from build123d import *

# Parameters (mm, degrees)
CROQUIS1_R              = 3.125
CROQUIS1_R_2            = 2.7
SALIENTE_EXTRUIR1_DEPTH = 10
CROQUIS2_W              = 22
CROQUIS2_H              = 15
SALIENTE_EXTRUIR2_DEPTH = 50
CROQUIS3_R              = 4
CORTAR_EXTRUIR1_DEPTH   = 63.841873384


with BuildPart() as part:
    # Croquis1 → Saliente-Extruir1 (new body)
    with BuildSketch(Plane.XY):
        with Locations((0.140065102, 8.039289834)):
            Circle(CROQUIS1_R)
        with Locations((0.140065102, 8.039289834)):
            Circle(CROQUIS1_R_2, mode=Mode.SUBTRACT)
    extrude(amount=SALIENTE_EXTRUIR1_DEPTH)

    # Croquis2 → Saliente-Extruir2 (add)
    with BuildSketch(Plane.XY.offset(10)):
        with Locations((0.140065102, 8.039289834)):
            Rectangle(CROQUIS2_W, CROQUIS2_H)
    extrude(amount=SALIENTE_EXTRUIR2_DEPTH)

    # Croquis3 → Cortar-Extruir1 (cut, through all)
    with BuildSketch(Plane.XZ.offset(-0.539289834)):
        with Locations(Location((0.140065102, 35, 0), (0, 0, 270))):
            Circle(CROQUIS3_R)
    extrude(amount=-CORTAR_EXTRUIR1_DEPTH, mode=Mode.SUBTRACT)


solid = part.part
Geometry check sheet. Reference: the model listing, model coordinates, mm. A direction names the side the tool comes from. Coordinates: 2 decimals unless noted, no trailing zeros. Order: outer loops, then holes, each group sorted by start corner. A loop starts at its lowest first (then second) coordinate and runs counter-clockwise, first axis right, second up. Notation, with made-up numbers: (44.5, 39) - (59.5, 39) arc R16 ccw to (59.5, 43) - close; hole circle Ø11 at (43, 27). An arc over 180 degrees is marked (long way). Answer in a Markdown table with one row per item. Add a question column.
1) Cross-section at D-D, the plane y = 8.75. Record the cut outline in (x, z), then the cut area to 3 significant figures.
2) Release check for a two-part mould opening along Y. For faces 3 (the flat face through (-5, 0.539, 35)), 4 (the cylindrical face through (-0.445, 5.403, 4.93)), 5 (the flat face through (0, 8, 10)), 6 (the flat face through (-5, 15.539, 35)) record: +Y half, -Y half, draft (parallel to the pull), parting line (faces both ways), or undercut.
3) Set-up check for faces 1 (the flat face through (11.14, 8, 35)), 2 (the flat face through (0, 11.5, 10)): record each of +Z, -Z, +X, -X, +Y, -Y from which the full face is reachable in a straight line by a thin tool's end or side.
4) Material ranges on line 1 along Z through (x, y) = (0, 14); line 2 along X through (y, z) = (7.75, 35); line 3 along Z through (x, y) = (7, 5), recorded low to high. Write a range as [from, to].
5) Cross-section at B-B, the plane y = 13.5. Record the cut outline in (x, z), then the cut area to 3 significant figures.
6) Cross-section at A-A, the plane z = 35. Record the cut outline in (x, y).
7) Cross-section at C-C, the plane x = 6.5. Record the cut outline in (y, z).
Check result:
| question | item | result |
|---|---|---|
| 1 | outline | (-10.86, 10) - (-2.9, 10) - (-2.9, 0) - (-2.46, 0) - (-2.46, 10) - (2.74, 10) - (2.74, 0) - (3.18, 0) - (3.18, 10) - (11.14, 10) - (11.14, 60) - (-10.86, 60) - close; hole circle Ø8 at (0.14, 35) |
| 1 | area | 1,060 mm² |
| 2 | face 3 | -Y half |
| 2 | face 4 | undercut |
| 2 | face 5 | undercut |
| 2 | face 6 | +Y half |
| 3 | face 1 | +Z, -Z, +X, +Y, -Y |
| 3 | face 2 | -Z |
| 4 | line 1 | z = [10, 31], [39, 60] |
| 4 | line 2 | x = [-10.86, -3.86], [4.14, 11.14] |
| 4 | line 3 | z = [10, 60] |
| 5 | outline | (-10.86, 10) - (11.14, 10) - (11.14, 60) - (-10.86, 60) - close; hole circle Ø8 at (0.14, 35) |
| 5 | area | 1,050 mm² |
| 6 | outline | (-10.86, 0.54) - (-3.86, 0.54) - (-3.86, 15.54) - (-10.86, 15.54) - close; (4.14, 0.54) - (11.14, 0.54) - (11.14, 15.54) - (4.14, 15.54) - close |
| 7 | outline | (0.54, 10) - (15.54, 10) - (15.54, 60) - (0.54, 60) - close |
